```python
from build123d import *

# Parameters (mm, degrees)
F0_R     = 15.875
F1_DEPTH = 47.625


with BuildPart() as f1:
    # F0 (on Front) → F1 (new body)
    with BuildSketch(Plane.XZ):
        with BuildLine():
            ThreePointArc((-65.487075, 63.5), (-97.237075, 31.75), (-65.487075, 0))
            Line((-65.487075, 0), (36.112925, 0))
            Line((36.112925, 0), (36.112925, 31.75))
            ThreePointArc((36.112925, 31.75), (13.662285, 41.04936), (4.362925, 63.5))
            Line((4.362925, 63.5), (-65.487075, 63.5))
        make_face()
        with Locations((-65.487075, 31.75)):
            Circle(F0_R, mode=Mode.SUBTRACT)
    extrude(amount=F1_DEPTH)


solid = f1.part
```
The listing builds one solid part. Answer for the finished solid, in the listing's coordinates (mm). Coordinates: 2 decimals unless noted, no trailing zeros. Write each loop counter-clockwise with the first axis right and the second up, starting at its lowest first coordinate (ties: lowest second). Pieces come first, ordered by that corner, then holes. Notation, with made-up numbers: M -4.5,20 L 20.5,20 A5 ccw 20.5,24 Z; hole C 74.5,-23.75 d10. An arc over 180 degrees is marked long. Use a Markdown table: item, result. Add a question column.
1. For a pull along Z with two mould halves and no side action, classify faces 1 (the flat face through (-30, -23, 63.5)), 2 (the flat face through (-31, -47.625, 32)), 3 (the cylindrical face through (-50.823, -23.479, 25.67)) as +Z half, -Z half, draft (parallel to the pull), parting line (faces both ways), or undercut.
2. Given P1, Ø1.5, axis at y = -41, z = 56.5, coming from the -X side; P2, Ø4, axis at x = 12.5, y = -36.5, coming from the +Z side; P3, Ø1, axis at y = -33, z = 46.5, coming from the +X side, each flat-ended and moving along its own axis, determine where each tip first touches the part or whether it passes through.
3. Straight lines are drawn through the part: line 1 along X through (y, z) = (-12, 31); line 2 along X through (y, z) = (-22.5, 40.5); line 3 along Z through (x, y) = (-75, -7.5). For each, find the intervals that lie inside material, in ascending order. Write a range as [from, to].
4. Section B-B (x = -62.5) is taken. Give the vertices of the cut face in (y, z) (3 decimals).
5. Section A-A (z = 36) is taken. Give the vertices of the cut face in (x, y) (3 decimals).
6. Section C-C (y = -36.5) is taken. Give the vertices of the cut face in (x, z) (3 decimals), plus the area to 3 significant figures.
7. Section D-D (x = 20.5) is taken. Give the vertices of the cut face in (y, z) (3 decimals).
Data:
| question | item | result |
|---|---|---|
| 1 | face 1 | +Z half |
| 1 | face 2 | draft |
| 1 | face 3 | undercut |
| 2 | P1 | stops at x = -86.27 |
| 2 | P2 | stops at z = 44.74 |
| 2 | P3 | stops at x = 9.62 |
| 3 | line 1 | x = [-97.23, -81.34], [-49.63, 36.11] |
| 3 | line 2 | x = [-96.01, -78.73], [-52.24, 14.23] |
| 3 | line 3 | z = [1.46, 19.04], [44.46, 62.04] |
| 4 | outline | M -47.625,0 L 0,0 L 0,16.159 L -47.625,16.159 Z; M -47.625,47.341 L 0,47.341 L 0,63.5 L -47.625,63.5 Z |
| 5 | outline | M -96.951,-47.625 L -80.783,-47.625 L -80.783,0 L -96.951,0 Z; M -50.192,-47.625 L 20.244,-47.625 L 20.244,0 L -50.192,0 Z |
| 6 | outline | M -65.487,0 L 36.113,0 L 36.113,31.75 A31.75 cw 4.363,63.5 L -65.487,63.5 A31.75 ccw Z; hole C -65.487,31.75 d31.75 |
| 6 | area | 6,450 mm2 |
| 7 | outline | M -47.625,0 L 0,0 L 0,35.854 L -47.625,35.854 Z |
